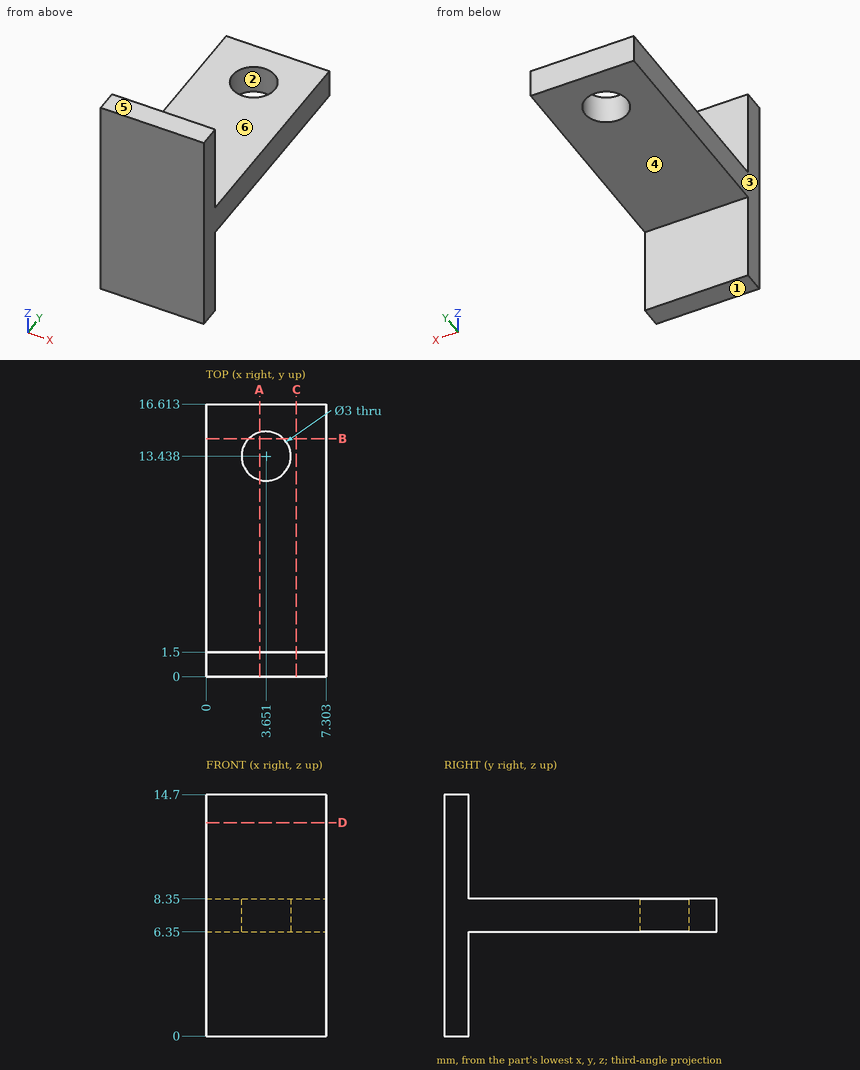
For this review, use the dimensioned drawing (mm, ordinates from the lowest corner) and the shaded views. A direction names the side the tool comes from. Round coordinates to 2 decimals unless told otherwise and drop trailing zeros. Loops run counter-clockwise (first coordinate to the right, second up) from the corner with the lowest first, then second, coordinate; pieces in that order, holes last. Notation, with made-up numbers: (29, 69) -> (52, 69) arc R34 ccw to (52, 102) -> close; hole circle Ø2 at (78, 15). An arc over 180 degrees is marked (long way). Write item = value, one per line. Start each with the question number.
Item 1: Take a section at C-C on x = 5.5. Give the boundary of the cut face in (y, z).
Item 2: Insertion check: pin 1 (2 mm diameter, centred on x = 3, y = 6.5, fed in from +Z); pin 2 (1.9 mm diameter, centred on x = 4, z = 10.5, fed in from +Y); pin 3 (3.5 mm diameter, centred on x = 3.65, y = 13.44, fed in from -Z); pin 4 (5 mm diameter, centred on y = 7, z = 2.5, fed in from +X). Each pin has a flat end and moves straight along its axis. Give the tip position at first contact, or say it passes through.
Item 3: Take a section at B-B on y = 14.5. Give the boundary of the cut face in (x, z).
Item 4: Mouldability with a two-part tool opening along X and no side actions: class the marked faces 1, 2 and 3 as released by +X, released by -X, zero draft, split by the parting line, or undercut.
Item 5: For the marked faces 4, 5 and 6, list the 3-axis set-ups (+Z, -Z, +X, -X, +Y, -Y) from which the entire face can be reached by the end or side of a thin tool; tool diameter is ignored.
Item 6: Take a section at D-D on z = 13. Give the boundary of the cut face in (x, y).
Item 7: Take a section at A-A on x = 3.25. Give the boundary of the cut face in (y, z).
Item 8: To check wall thickness, follow L1, parallel to Y at x = 0.75, z = 0.5; L2, parallel to Z at x = 6.75, y = 10.25; L3, parallel to Y at x = 4, z = 6.75. State the ranges of each line that lie inside material, in increasing order.
Result:
q1.outline = (0, 0) -> (1.5, 0) -> (1.5, 6.35) -> (16.61, 6.35) -> (16.61, 8.35) -> (1.5, 8.35) -> (1.5, 14.7) -> (0, 14.7) -> close
q2.pin_1 = 8.35
q2.pin_2 = 1.5
q2.pin_3 = 6.35
q2.pin_4 = through
q3.outline = (0, 6.35) -> (2.59, 6.35) -> (2.59, 8.35) -> (0, 8.35) -> close; (4.71, 6.35) -> (7.3, 6.35) -> (7.3, 8.35) -> (4.71, 8.35) -> close
q4.face_1 = zero draft
q4.face_2 = undercut
q4.face_3 = released by -X
q5.face_4 = -Z, +X, -X, +Y
q5.face_5 = +Z, +X, -X, +Y, -Y
q5.face_6 = +Z, +X, -X, +Y
q6.outline = (0, 0) -> (7.3, 0) -> (7.3, 1.5) -> (0, 1.5) -> close
q7.outline = (0, 0) -> (1.5, 0) -> (1.5, 6.35) -> (11.99, 6.35) -> (11.99, 8.35) -> (1.5, 8.35) -> (1.5, 14.7) -> (0, 14.7) -> close; (14.88, 6.35) -> (16.61, 6.35) -> (16.61, 8.35) -> (14.88, 8.35) -> close
q8.L1 = 0 to 1.5
q8.L2 = 6.35 to 8.35
q8.L3 = 0 to 11.98, 14.9 to 16.61
